from build123d import *

# Parameters (mm, degrees)
SALIENTE_EXTRUIR1_DEPTH = 25
CROQUIS6_R              = 2.7
CORTAR_EXTRUIR1_DEPTH   = 15
CROQUIS7_R              = 8.4
CORTAR_EXTRUIR2_DEPTH   = 10


with BuildPart() as part:
    # Croquis1 → Saliente-Extruir1 (new, symmetric)
    with BuildSketch(Plane(origin=(0, 0, 0), x_dir=(1, 0, 0), z_dir=(0, 1, 0))):
        Polygon((-28.867513459, 0), (28.867513459, 0), (0, -50), align=None)
    extrude(amount=SALIENTE_EXTRUIR1_DEPTH, both=True)

    # Croquis6 → Cortar-Extruir1 (cut, symmetric)
    with BuildSketch(Plane.XY):
        with Locations((-23.070667369, 0)):
            Circle(CROQUIS6_R)
        with Locations(Location((23.082974371, 9.835520027, 0), (0, 0, 180))):
            Circle(CROQUIS6_R)
    extrude(amount=CORTAR_EXTRUIR1_DEPTH, both=True, mode=Mode.SUBTRACT)

    # Croquis7 → Cortar-Extruir2 (cut)
    with BuildSketch(Plane(origin=(0, 0, 6), x_dir=(-1, 0, 0), z_dir=(0, 0, -1))):
        with Locations((-23.082974371, 9.835520027)):
            Circle(CROQUIS7_R)
        with Locations((23.070667369, 0)):
            Circle(CROQUIS7_R)
    extrude(amount=-CORTAR_EXTRUIR2_DEPTH, mode=Mode.SUBTRACT)


solid = part.part
Source: CAD feature listing. Evaluate the final solid. Frame: model axes, mm. A direction names the side the tool comes from. Round coordinates to 2 decimals unless told otherwise and drop trailing zeros. Loops run counter-clockwise (first coordinate to the right, second up) from the corner with the lowest first, then second, coordinate; pieces in that order, holes last. Notation, with made-up numbers: M -39.5,26 L -3.5,26 A26 ccw -3.5,53 Z; hole C -21,60.25 d4. An arc over 180 degrees is marked long. Return JSON: item names as keys, results as strings. Group by question number.
1. Material intervals for line 1 along X through (y, z) = (-10, 16); line 2 along X through (y, z) = (1, 26); line 3 along Z through (x, y) = (14, -14), sorted ascending. Write a range as from..to.
2. Mould query, pull axis Y, two halves, no side actions, for faces 1 (the face through (0, 25, 19)), 2 (the face through (18, 10, 16)), 3 (the face through (0, 0, 0)). Classes: released by +Y, released by -Y, zero draft, split by the parting line, or undercut.
3. Reachability of faces 4 (the face through (-18, 0, 16)), 5 (the face through (0, -25, 19)) from +Z, -Z, +X, -X, +Y, -Y: full face, straight path, thin tool, end or side. Return the list, or none.
4. Section query A-A on y = 0. Output: boundary loops of the cut face in (x, z), and give its area (3 significant figures).
5. Section query D-D on x = -3.5. Output: boundary loops of the cut face in (y, z).
6. Pin query (flat end, axial travel): pin 1 (1 mm diameter, centred on x = -12.5, y = -3, fed in from +Z); pin 2 (3 mm diameter, centred on x = -23.07, y = 0, fed in from +Z); pin 3 (13.5 mm diameter, centred on x = -23.07, y = 0, fed in from +Z); pin 4 (1.5 mm diameter, centred on y = -19, z = 5.5, fed in from +X). Return the tip coordinate at first contact, or that it passes through.
7. Section query C-C on z = 31. Output: boundary loops of the cut face in (x, y).
8. Section query B-B on y = -14. Output: boundary loops of the cut face in (x, z), and give its area (3 significant figures).
Checks:
{
 "1": {"line 1": "x = -19.63..19.63", "line 2": "x = -13.86..13.86", "line 3": "z = 0..25.75"},
 "2": {"face 1": "released by +Y", "face 2": "undercut", "face 3": "zero draft"},
 "3": {"face 4": "-X", "face 5": "+Z, -Z, +X, -X, -Y"},
 "4": {"outline": "M -28.87,0 L -25.77,0 L -25.77,5.36 Z; M -20.37,0 L 28.87,0 L 0,50 L -19.63,16 L -14.67,16 L -14.67,6 L -20.37,6 Z", "area": "1,330 mm²"},
 "5": {"outline": "M -25,0 L 25,0 L 25,43.94 L -25,43.94 Z"},
 "6": {"pin 1": "stops at z = 29.22", "pin 2": "passes through", "pin 3": "stops at z = 21.73", "pin 4": "stops at x = 26.13"},
 "7": {"outline": "M -10.97,-25 L 10.97,-25 L 10.97,25 L -10.97,25 Z"},
 "8": {"outline": "M -28.87,0 L 28.87,0 L 0,50 Z", "area": "1,440 mm²"}
}
